```python
from build123d import *

# Parameters (mm, degrees)
F0_R     = 11.2
F1_DEPTH = 7


with BuildPart() as f1:
    # F0 (on Top) → F1 (new body)
    with BuildSketch(Plane.XY):
        with BuildLine():
            ThreePointArc((2.687978, -12.92342), (10.240149, -8.329427), (13.2, 0))
            ThreePointArc((13.2, 0), (12.970512, 2.450679), (12.290026, 4.816146))
            ThreePointArc((12.290026, 4.816146), (11.245901, 6.911563), (9.848021, 8.789567))
            ThreePointArc((9.848021, 8.789567), (-0.32942, 13.195889), (-10.274323, 8.287236))
            ThreePointArc((-10.274323, 8.287236), (-11.601306, 6.296801), (-12.547257, 4.099555))
            ThreePointArc((-12.547257, 4.099555), (-11.23644, -6.926934), (-1.974108, -13.051548))
            ThreePointArc((-1.974108, -13.051548), (0.362639, -13.195018), (2.687978, -12.92342))
        make_face()
        Circle(F0_R, mode=Mode.SUBTRACT)
        with BuildLine():
            ThreePointArc((12.290026, 4.816146), (12.970512, 2.450679), (13.2, 0))
            ThreePointArc((13.2, 0), (10.240149, -8.329427), (2.687978, -12.92342))
            ThreePointArc((2.687978, -12.92342), (7.094996, -14.488543), (10.640132, -17.538696))
            Line((10.640132, -17.538696), (11.942446, -19.917944))
            Line((11.942446, -19.917944), (14.567682, -24.714088))
            Line((14.567682, -24.714088), (25.063097, -27.784215))
            Line((25.063097, -27.784215), (34.655385, -22.533744))
            Line((34.655385, -22.533744), (37.725512, -12.038328))
            Line((37.725512, -12.038328), (32.475041, -2.446041))
            Line((32.475041, -2.446041), (21.979625, 0.624087))
            ThreePointArc((21.979625, 0.624087), (16.680073, 1.668994), (12.290026, 4.816146))
        make_face()
        with Locations((23.521361, -13.580064)):
            Circle(F0_R, mode=Mode.SUBTRACT)
        with BuildLine():
            ThreePointArc((-10.274323, 8.287236), (-0.32942, 13.195889), (9.848021, 8.789567))
            ThreePointArc((9.848021, 8.789567), (9.000749, 13.505555), (9.955713, 18.20092))
            Line((9.955713, 18.20092), (13.510024, 22.219826))
            Line((13.510024, 22.219826), (12.840438, 33.134545))
            Line((12.840438, 33.134545), (4.649097, 40.378947))
            Line((4.649097, 40.378947), (-6.265622, 39.709361))
            Line((-6.265622, 39.709361), (-13.510024, 31.51802))
            Line((-13.510024, 31.51802), (-12.840438, 20.603301))
            ThreePointArc((-12.840438, 20.603301), (-9.935568, 14.783181), (-10.274323, 8.287236))
        make_face()
        with Locations((0, 26.868923)):
            Circle(F0_R, mode=Mode.SUBTRACT)
        with BuildLine():
            ThreePointArc((-12.732913, -19.541365), (-8.20936, -14.877632), (-1.974108, -13.051548))
            ThreePointArc((-1.974108, -13.051548), (-11.23644, -6.926934), (-12.547257, 4.099555))
            ThreePointArc((-12.547257, 4.099555), (-16.453714, 0.896577), (-21.29652, -0.541025))
            ThreePointArc((-21.29652, -0.541025), (-21.351853, -0.545868), (-21.407206, -0.550469))
            ThreePointArc((-21.407206, -0.550469), (-21.775008, -0.496095), (-22.144195, -0.452101))
            Line((-22.144195, -0.452101), (-26.19324, -0.027343))
            Line((-26.19324, -0.027343), (-27.581975, 0.11834))
            Line((-27.581975, 0.11834), (-36.078883, -6.765118))
            Line((-36.078883, -6.765118), (-37.219765, -17.640678))
            Line((-37.219765, -17.640678), (-30.336308, -26.137586))
            Line((-30.336308, -26.137586), (-19.460747, -27.278468))
            Line((-19.460747, -27.278468), (-12.732913, -19.541365))
        make_face()
        with Locations((-23.26917, -13.725667)):
            Circle(F0_R, mode=Mode.SUBTRACT)
        with BuildLine():
            ThreePointArc((-21.407206, -0.550469), (-21.351853, -0.545868), (-21.29652, -0.541025))
            Line((-21.29652, -0.541025), (-22.144195, -0.452101))
            ThreePointArc((-22.144195, -0.452101), (-21.775008, -0.496095), (-21.407206, -0.550469))
        make_face()
    extrude(amount=F1_DEPTH)


solid = f1.part
```
Here's how the part is built. I have some questions about the finished solid (model axes, mm). A direction names the side the tool comes from. Coordinates: 2 decimals unless noted, no trailing zeros. Order: outer loops, then holes, each group sorted by start corner. A loop starts at its lowest first (then second) coordinate and runs counter-clockwise, first axis right, second up.
Item 1: If we section it at C-C, the plane x = 1: List the corners of the cut face in (y, z) for me, then the cut area to 3 significant figures.
Response values:
outline: (-13.16, 0) - (-11.16, 0) - (-11.16, 7) - (-13.16, 7) - close; (11.16, 0) - (15.71, 0) - (15.71, 7) - (11.16, 7) - close; (38.02, 0) - (40.16, 0) - (40.16, 7) - (38.02, 7) - close
area: 60.9 mm2
Item 2: Thinking about a two-plate mould opening in Y: for faces 1 (the face through (0.33, -13.196, 3.451)), 2 (the face through (-13.18, 26.14, 3.45)), 3 (the face through (8.8, 36.71, 3.45)), which applies, pulls with the +Y half, pulls with the -Y half, needs draft (parallel to the pull), parting line crosses it, or undercut?
Response values:
face 1: pulls with the -Y half
face 2: undercut
face 3: pulls with the +Y half
Item 3: If we section it at A-A, the plane x = -16: List the corners of the cut face in (y, z) for me, then the cut area to 3 significant figures.
Response values:
outline: (-23.3, 0) - (-22.25, 0) - (-22.25, 7) - (-23.3, 7) - close; (-5.21, 0) - (1.15, 0) - (1.15, 7) - (-5.21, 7) - close
area: 51.8 mm2
Item 4: I need wall thicknesses on probe 1 along X at (y, z) = (-20, 4.5); probe 2 along X at (y, z) = (-7.5, 6.5); probe 3 along Y at (x, z) = (-3.5, 3.75). Which ranges of each line are inside material? Lowest first, please.
Response values:
probe 1: x = -35.31 to -32.55, -13.99 to -13.13, 11.99 to 14.34, 32.7 to 35.4
probe 2: x = -36.16 to -32.58, -13.96 to -8.32, 8.32 to 14.12, 32.93 to 35.24
probe 3: y = -13.18 to -10.64, 10.64 to 16.23, 37.51 to 39.88
Item 5: I'm going to push flat-ended pins straight in: pin 1 Ø1 at (y, z) = (27.5, 2.5) entering from -X; pin 2 Ø3 at (x, z) = (-12, 2.5) entering from -Y; pin 3 Ø1.5 at (x, z) = (28, 2.5) entering from +Y. Where does each tip first touch, or does it pass through?
Response values:
pin 1: stops at x = -13.29
pin 2: stops at y = -20.42
pin 3: stops at y = -0.92
Item 6: Which directions (+Z, -Z, +X, -X, +Y, -Y) give clear straight access to the entire face, cutting with the end or side of a thin tool? Please do faces 4 (the face through (7.038, -14.456, 3.451)), 5 (the face through (-11.19, 0.49, 3.45)), 6 (the face through (11.708, 20.182, 3.451)).
Response values:
face 4: +Z, -Z, -Y
face 5: +Z, -Z
face 6: +Z, -Z, +X
Item 7: If we section it at B-B, the plane y = 25: List the corners of the cut face in (x, z) for me, then the cut area to 3 significant figures.
Response values:
outline: (-13.11, 0) - (-11.04, 0) - (-11.04, 7) - (-13.11, 7) - close; (11.04, 0) - (13.34, 0) - (13.34, 7) - (11.04, 7) - close
area: 30.5 mm2
